from build123d import *

# Parameters (mm, degrees)
CYLINDER003_R          = 20
CYLINDER003_DEPTH      = 116
CYLINDER004_R          = 20
CYLINDER004_DEPTH      = 55
FUSION_PLACEMENT_ANGLE = 90


with BuildPart() as cylinder:
    # Cylinder003 → Cylinder003 (new body)
    with BuildSketch(Plane.XY):
        Circle(CYLINDER003_R)
    extrude(amount=CYLINDER003_DEPTH)


with BuildPart() as obj1:
    # Cylinder004 → Cylinder004 (new body)
    with BuildSketch(Plane(origin=(0, 0, 58), x_dir=(0, 0, -1), z_dir=(1, 0, 0))):
        Circle(CYLINDER004_R)
    extrude(amount=CYLINDER004_DEPTH)

    # Fusion: union Cylinder
    add(cylinder.part)


with BuildPart() as obj1_1:
    # Fusion placement: moved
    add(obj1.part.moved(Location((450, -120, -550))).rotate(Axis((450, -120, -550), (0, 1, 0)), FUSION_PLACEMENT_ANGLE))


solid = obj1_1.part
The listing builds one solid part. Answer for the finished solid, in the listing's coordinates (mm). A direction names the side the tool comes from. Coordinates: 2 decimals unless noted, no trailing zeros. Loops run counter-clockwise (first coordinate to the right, second up) from the corner with the lowest first, then second, coordinate; pieces in that order, holes last. Notation, with made-up numbers: (-31.75, 71.5) -> (2.25, 71.5) arc R16 cw to (2.25, 78.5) -> close; hole circle Ø3 at (-28, 61). An arc over 180 degrees is marked (long way). Answer in a Markdown table with one row per item. Add a question column.
1. The part is cut by section D-D, the plane y = -132. Write down the section's boundary in (x, z), then the cut area to 3 significant figures.
2. For faces 1 (the cylindrical face through (510.6, -100.17, -583.23)), 2 (the flat face through (450, -120, -550)), 3 (the cylindrical face through (507.19, -119.12, -530.02)), determine the directions among +Z, -Z, +X, -X, +Y, -Y from which every point of the face is accessible in a straight line to the end or side of a thin tool.
3. The part is cut by section B-B, the plane z = -538. Write down the section's boundary in (x, y).
4. Consider line 1 (Z direction, x = 490, y = -119); line 2 (Y direction, x = 502.5, z = -586.5); line 3 (Z direction, x = 462, y = -108.5). Determine where each line is inside the solid, lowest interval first. Write a range as [from, to].
5. Flat-ended cylindrical pins translate along their axes: P1, Ø6, axis at y = -127.5, z = -588, coming from the +X side; P2, Ø3, axis at y = -131.5, z = -569.5, coming from the +X side; P3, Ø8, axis at x = 485, y = -130.5, coming from the -Z side. Find the tip coordinate at first contact, or state that the pin passes through.
6. The part is cut by section C-C, the plane x = 508. Write down the section's boundary in (y, z).
7. The part is cut by section A-A, the plane y = -120. Write down the section's boundary in (x, z), then the cut area to 3 significant figures.
Answer below:
| question | item | result |
|---|---|---|
| 1 | outline | (450, -566) -> (492, -566) -> (492, -605) -> (524, -605) -> (524, -566) -> (566, -566) -> (566, -534) -> (450, -534) -> close |
| 1 | area | 4,960 mm2 |
| 2 | face 1 | -Z |
| 2 | face 2 | +Z, -Z, -X, +Y, -Y |
| 2 | face 3 | none |
| 3 | outline | (450, -136) -> (566, -136) -> (566, -104) -> (450, -104) -> close |
| 4 | line 1 | [-605, -530.03] |
| 4 | line 2 | [-139.23, -100.77] |
| 4 | line 3 | [-566.36, -533.64] |
| 5 | P1 | x = 527.49 |
| 5 | P2 | x = 525.32 |
| 5 | P3 | z = -568.91 |
| 6 | outline | (-140, -605) -> (-100, -605) -> (-100, -550) arc R20 ccw to (-140, -550) -> close |
| 7 | outline | (450, -570) -> (488, -570) -> (488, -605) -> (528, -605) -> (528, -570) -> (566, -570) -> (566, -530) -> (450, -530) -> close |
| 7 | area | 6,040 mm2 |
